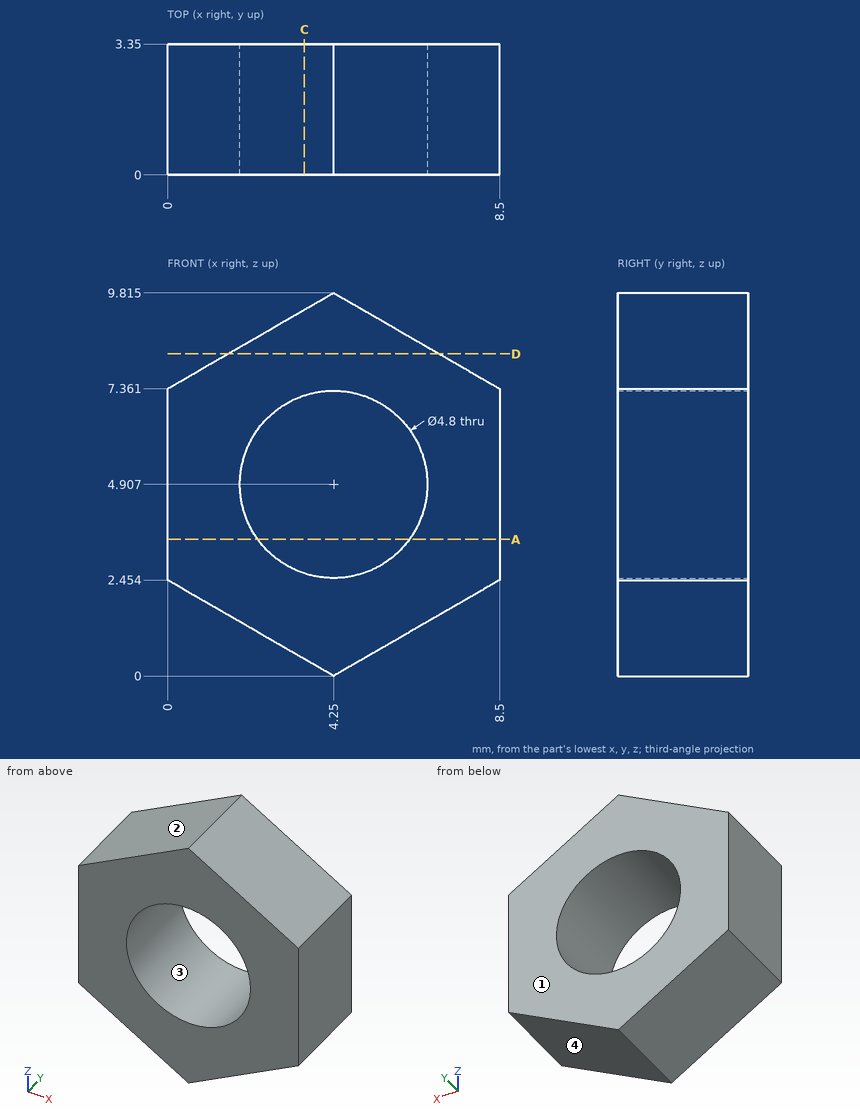
Geometry check sheet. Reference: drawing and pictorial views, mm from the part's lowest x, y, z. Coordinates: 2 decimals unless noted, no trailing zeros. Order: outer loops, then holes, each group sorted by start corner. A loop starts at its lowest first (then second) coordinate and runs counter-clockwise, first axis right, second up. Notation, with made-up numbers: (43.5, 19) -> (88.5, 19) arc R20 cw to (88.5, 29) -> close; hole circle Ø3 at (27, 82). An arc over 180 degrees is marked (long way). Write item = value, one per line. Start each with the question number.
1) Mould release check, pull along X, two halves, no side actions. Record for the marked faces 1, 2, 3 and 4: +X half, -X half, draft (parallel to the pull), parting line (faces both ways), or undercut.
2) Cross-section at D-D (z = 8.25). Enter the section's corners in (x, y).
3) Cross-section at A-A (z = 3.5). Enter the section's corners in (x, y).
4) Go/stop test with a flat-tipped pin: P1, Ø2, axis at x = 7, y = 2.5, coming from the -Z side. Record where the tip stops, or that it passes through.
5) Material ranges on L1, parallel to X at y = 2.1, z = 5; L2, parallel to X at y = 1.05, z = 5.75; L3, parallel to Z at x = 2.25, y = 0.45 (1 decimal), recorded low to high.
6) Cross-section at C-C (x = 3.5). Enter the section's corners in (y, z), then the cut area to 3 significant figures.
Ans:
q1.face_1 = draft
q1.face_2 = -X half
q1.face_3 = undercut
q1.face_4 = +X half
q2.outline = (1.54, 0) -> (6.96, 0) -> (6.96, 3.35) -> (1.54, 3.35) -> close
q3.outline = (0, 0) -> (2.31, 0) -> (2.31, 3.35) -> (0, 3.35) -> close; (6.19, 0) -> (8.5, 0) -> (8.5, 3.35) -> (6.19, 3.35) -> close
q4.P1 = 1.01
q5.L1 = 0 to 1.85, 6.65 to 8.5
q5.L2 = 0 to 2, 6.5 to 8.5
q5.L3 = 1.2 to 3.6, 6.2 to 8.7
q6.outline = (0, 0.43) -> (3.35, 0.43) -> (3.35, 2.63) -> (0, 2.63) -> close; (0, 7.19) -> (3.35, 7.19) -> (3.35, 9.38) -> (0, 9.38) -> close
q6.area = 14.7 mm²
